The listing builds one solid part. Answer for the finished solid, in the listing's coordinates (mm). Round coordinates to 2 decimals unless told otherwise and drop trailing zeros. Loops run counter-clockwise (first coordinate to the right, second up) from the corner with the lowest first, then second, coordinate; pieces in that order, holes last. Notation, with made-up numbers: (12.25, 53) -> (31.25, 53) arc R23 cw to (31.25, 73) -> close; hole circle Ø9 at (25.5, 36.5). An arc over 180 degrees is marked (long way). Write each question's results on one line, items separated by ' | '. Start each with the question number.
from build123d import *

# Parameters (mm, degrees)
F0_R     = 3.937
F1_DEPTH = 50.8
F2_R     = 2.54
F3_DEPTH = 15.24
F6_SIZE  = 0.635


with BuildPart() as f1:
    # F0 (on Top) → F1 (new body)
    with BuildSketch(Plane.XY):
        Circle(F0_R)
    extrude(amount=F1_DEPTH)

    # F2 (on Right) → F3 (join)
    with BuildSketch(Plane.YZ):
        with Locations((0, 25.4)):
            Circle(F2_R)
    extrude(amount=F3_DEPTH)

    # F4 (on Front) → F5 (revolve)
    with BuildSketch(Plane.XZ):
        with BuildLine():
            add(Edge.make_bspline(
                [(18.9343895763, 28.8740284741), (17.7644916054, 29.4402146526), (15.5309316536, 30.5211728258), (11.5248021674, 29.2662104574), (12.2419333681, 26.7555454392), (12.6073630527, 25.4761818796)],
                knots=[0, 0, 0, 0, 0.350400992, 0.6689828021, 1, 1, 1, 1], degree=3))
            Line((12.6073630527, 25.4761818796), (18.9343895763, 25.4761818796))
            Line((18.9343895763, 25.4761818796), (18.9343895763, 28.8740284741))
        make_face()
    revolve(axis=Axis((15.24, 0, 25.4), (1, 0, 0)))

    # F6
    f6_edges = [f1.edges().sort_by_distance(p)[0] for p in [
        (-3.937, 0, 50.8),
        (-3.937, 0, 0),
    ]]
    chamfer(f6_edges, length=F6_SIZE)


solid = f1.part
Item 1: Each of these flat-tipped pins is pushed along its axis until it touches: pin 1 Ø4 at (x, y) = (14.5, 2) entering from -Z; pin 2 Ø1.5 at (y, z) = (3.5, 42) entering from -X; pin 3 Ø1 at (y, z) = (-2.5, 22.5) entering from -X. Where does it stop, or does it pass through?
Item 2: Straight lines are drawn through the part: L1, parallel to Z at x = 17.75, y = 0; L2, parallel to Z at x = 16.05, y = 0; L3, parallel to X at y = 3, z = 23. For each, find the intervals that lie inside material, in ascending order. Write a range as [from, to].
Item 3: The part is cut by section A-A, the plane x = 0. Give the vertices of the cut face in (y, z) (3 decimals).
Item 4: Determine the mould class of faces 1 (the cylindrical face through (7.506, 1.172, 23.147)), 2 (the flat face through (0, 0, 0)), 3 (the flat face through (18.934, 0, 25)) for opening direction X: +X half, -X half, draft (parallel to the pull), parting line (faces both ways), or undercut.
Report:
1) pin 1: stops at z = 20.75 | pin 2: stops at x = -2.82 | pin 3: stops at x = -3.39
2) L1: z = [21.38, 25.32], [25.48, 29.42] | L2: z = [20.83, 25.32], [25.48, 29.97] | L3: x = [-2.55, 2.55], [12.67, 18.16]
3) outline: (-3.937, 0.635) -> (-3.302, 0) -> (3.302, 0) -> (3.937, 0.635) -> (3.937, 50.165) -> (3.302, 50.8) -> (-3.302, 50.8) -> (-3.937, 50.165) -> close
4) face 1: undercut | face 2: draft | face 3: +X half
